```python
from build123d import *

# Parameters (mm, degrees)
F2_SIZE  = 1
F3_R     = 3
F4_DEPTH = 25


with BuildPart() as f1:
    # F0 (on Front) → F1 (revolve)
    with BuildSketch(Plane.XZ):
        with BuildLine():
            Line((-36, 0), (-20.05, 0))
            Line((-20.05, 0), (-20.05, 8))
            Line((-20.05, 8), (-26.5, 8))
            ThreePointArc((-26.5, 8), (-40.288582, 13.711418), (-46, 27.5))
            ThreePointArc((-46, 27.5), (-48.5, 30), (-51, 27.5))
            ThreePointArc((-51, 27.5), (-47.657601, 15.146623), (-38.542373, 6.163851))
            ThreePointArc((-38.542373, 6.163851), (-36.682122, 4.330632), (-36, 1.809535))
            Line((-36, 1.809535), (-36, 0))
        make_face()
    revolve(axis=Axis((0, 0, 4), (0, 0, 1)))

    # F2
    f2_edges = [f1.edges().sort_by_distance(p)[0] for p in [
        (20.05, 0, 0),
    ]]
    chamfer(f2_edges, length=F2_SIZE)

    # F3 (on Top) → F4 (cut)
    with BuildSketch(Plane.XY):
        with Locations((-28, 0)):
            Circle(F3_R)
        with Locations((0, 28)):
            Circle(F3_R)
        with Locations((28, 0)):
            Circle(F3_R)
        with Locations((0, -28)):
            Circle(F3_R)
    extrude(amount=F4_DEPTH, mode=Mode.SUBTRACT)


solid = f1.part
```
Could you check a few things on this model? Use its own coordinates, in mm. Round coordinates to 2 decimals unless told otherwise and drop trailing zeros. Loops run counter-clockwise (first coordinate to the right, second up) from the corner with the lowest first, then second, coordinate; pieces in that order, holes last. Notation, with made-up numbers: (-38.75, 25.5) - (-20.75, 25.5) arc R21 cw to (-20.75, 35.5) - close; hole circle Ø7 at (27, -21.5). An arc over 180 degrees is marked (long way). Answer in a Markdown table with one row per item. Add a question column.
(1) If we section it at A-A (y = 0): Please give me the cut outline in (x, z), plus the area to 3 significant figures.
(2) If we mould it in two halves opening along Y, with no side actions, what happens to faces 1 (the face through (17, 11, 8)), 2 (the face through (4.686, -35.694, 0.892)), 3 (the face through (-15, 15, 0))? For each: pulls with the +Y half, pulls with the -Y half, needs draft (parallel to the pull), parting line crosses it, or undercut.
(3) I need wall thicknesses on line 1 along X through (y, z) = (0, 5); line 2 along X through (y, z) = (0, 3); line 3 along Y through (x, z) = (0, 3.5). Which ranges of each line are inside material? Lowest first, please.
(4) I'm going to push flat-ended pins straight in: pin 1 (3 mm diameter, centred on x = 2, z = 3.5, fed in from -Y); pin 2 (2 mm diameter, centred on x = 24, z = 16.5, fed in from -Y); pin 3 (10 mm diameter, centred on y = 28, z = 13, fed in from -X); pin 4 (12 mm diameter, centred on x = -21, y = -13, fed in from -Z). Where does each tip first touch, or does it pass through?
(5) If we section it at B-B (z = 15): Please give me the cut outline in (x, y), plus the area to 3 significant figures.
Model answer:
| question | item | result |
|---|---|---|
| 1 | outline | (-51, 27.5) arc R24.5 ccw to (-38.54, 6.16) arc R5 cw to (-36, 1.81) - (-36, 0) - (-31, 0) - (-31, 8.53) arc R19.5 cw to (-46, 27.5) arc R2.5 ccw to start; (-25, 0) - (-21.05, 0) - (-20.05, 1) - (-20.05, 8) - (-25, 8) - close; (20.05, 1) - (21.05, 0) - (25, 0) - (25, 8) - (20.05, 8) - close; (31, 0) - (36, 0) - (36, 1.81) arc R5 cw to (38.54, 6.16) arc R24.5 ccw to (51, 27.5) arc R2.5 ccw to (46, 27.5) arc R19.5 cw to (31, 8.53) - close |
| 1 | area | 442 mm² |
| 2 | face 1 | undercut |
| 2 | face 2 | parting line crosses it |
| 2 | face 3 | needs draft |
| 3 | line 1 | x = -37.15 to -31, -25 to -20.05, 20.05 to 25, 31 to 37.15 |
| 3 | line 2 | x = -36.14 to -31, -25 to -20.05, 20.05 to 25, 31 to 36.14 |
| 3 | line 3 | y = -36.29 to -31, -25 to -20.05, 20.05 to 25, 31 to 36.29 |
| 4 | pin 1 | stops at y = -37.1 |
| 4 | pin 2 | stops at y = -42.81 |
| 4 | pin 3 | stops at x = -41.77 |
| 4 | pin 4 | stops at z = 0 |
| 5 | outline | circle Ø95.14 at (0, 0); hole circle Ø82.93 at (0, 0) |
| 5 | area | 1,710 mm² |
